```python
from build123d import *

# Parameters (mm, degrees)
EXTRUDE_1_DEPTH      = 5
EXTRUDE_1_DEPTH_BACK = 5
SKETCH_1_R           = 26
SKETCH_1_R_2         = 22


with BuildPart() as part:
    # Sketch 1 → Extrude 1 (new, two sides: drawn at the far end of the back side and taken through both)
    with BuildSketch(Plane.XY.offset(-EXTRUDE_1_DEPTH_BACK)):
        Circle(SKETCH_1_R)
        Circle(SKETCH_1_R_2, mode=Mode.SUBTRACT)
    extrude(amount=EXTRUDE_1_DEPTH + EXTRUDE_1_DEPTH_BACK)

    # Sketch 5 → Revolve 2 (revolve)
    with BuildSketch(Plane(origin=(0, 0, 0), x_dir=(0, 0, -1), z_dir=(1, 0, 0)), mode=Mode.PRIVATE) as revolve_2_sk:
        Polygon((-3, 19.5), (3, 19.5), (4, 22), (-4, 22), align=None)
    revolve(revolve_2_sk.sketch.rotate(Axis((0, 0, 5), (0, 0, -1)), 90), axis=Axis((0, 0, 5), (0, 0, -1)))


solid = part.part
```
Model file for the job. Use its own axes, mm. A direction names the side the tool comes from. Coordinates: 2 decimals unless noted, no trailing zeros. Loops run counter-clockwise (first coordinate to the right, second up) from the corner with the lowest first, then second, coordinate; pieces in that order, holes last. Notation, with made-up numbers: (-17, -26) -> (41, -26) arc R15 ccw to (41, 1) -> close; hole circle Ø7 at (3, -32.5). An arc over 180 degrees is marked (long way). Answer as a JSON object with one key per item and string values.
Q1. 3-axis set-ups, long thin cutter, end or side, ignore diameter. For faces 5 (the cylindrical face through (-4.769, -21.477, 4.493)), 6 (the cylindrical face through (-2.539, -19.334, -0.042)): which of +Z, -Z, +X, -X, +Y, -Y reach the whole face in a straight line?
Report:
{"face 5": "+Z", "face 6": "+Z, -Z"}
Q2. Flat gauge pins, fed straight in: P1, Ø6, axis at y = -9, z = -0.5, coming from the -X side; P2, Ø4, axis at y = 9, z = 3, coming from the +X side; P3, Ø5, axis at x = 10.5, y = 15.5, coming from the -Z side. Where does each tip first touch, or does it go through?
Report:
{"P1": "stops at x = -25.3", "P2": "stops at x = 25.04", "P3": "stops at z = -3.69"}
Q3. Cut at C-C (z = 0). List the corners of the cut face in (x, y), and give its area (3 significant figures).
Report:
{"outline": "circle Ø52 at (0, 0); hole circle Ø39 at (0, 0)", "area": "929 mm2"}
Q4. Pull direction Y, two halves, no side cores. Call faces 1 (the cylindrical face through (-4.769, -21.477, -4.507)), 2 (the conical face through (18.749, -5.904, -3.063)), 3 (the flat face through (-19, 12, 5)), 4 (the cylindrical face through (-20.633, -15.821, -0.07)): released by +Y, released by -Y, zero draft, split by the parting line, or undercut.
Report:
{"face 1": "undercut", "face 2": "undercut", "face 3": "zero draft", "face 4": "split by the parting line"}
Q5. Probe probe 1 along Y at (x, z) = (0, -1.45); probe 2 along Y at (x, z) = (0, -4.7); probe 3 along X at (y, z) = (-17.5, -2.75). List the from-to ranges inside material, lowest first.
Report:
{"probe 1": "y = -26 to -19.5, 19.5 to 26", "probe 2": "y = -26 to -22, 22 to 26", "probe 3": "x = -19.23 to -8.6, 8.6 to 19.23"}
Q6. Cut at A-A (y = 0). List the corners of the cut face in (x, z).
Report:
{"outline": "(-26, -5) -> (-22, -5) -> (-22, -4) -> (-19.5, -3) -> (-19.5, 3) -> (-22, 4) -> (-22, 5) -> (-26, 5) -> close; (19.5, -3) -> (22, -4) -> (22, -5) -> (26, -5) -> (26, 5) -> (22, 5) -> (22, 4) -> (19.5, 3) -> close"}
